from build123d import *

# Parameters (mm, degrees)
SKETCH1_W           = 19.8
SKETCH1_H           = 28
BOSS_EXTRUDE1_DEPTH = 3.7
SKETCH2_W           = 19.8
SKETCH2_H           = 3.7
BOSS_EXTRUDE2_DEPTH = 24.3
CUT_EXTRUDE1_DEPTH  = 9
BOSS_EXTRUDE3_DEPTH = 3.3
BOSS_EXTRUDE4_DEPTH = 3.3
BOSS_EXTRUDE5_DEPTH = 2.1
BOSS_EXTRUDE6_DEPTH = 1.5


with BuildPart() as part:
    # Sketch1 → Boss-Extrude1 (new body)
    with BuildSketch(Plane.XY):
        with Locations((9.9, 14)):
            Rectangle(SKETCH1_W, SKETCH1_H)
        with BuildLine():
            Line((13.2, 15.7), (13.2, 12.3))
            ThreePointArc((13.2, 12.3), (9.9, 9), (6.6, 12.3))
            Line((6.6, 12.3), (6.6, 15.7))
            ThreePointArc((6.6, 15.7), (9.9, 19), (13.2, 15.7))
        make_face(mode=Mode.SUBTRACT)
    extrude(amount=BOSS_EXTRUDE1_DEPTH)

    # Sketch2 → Boss-Extrude2 (add)
    with BuildSketch(Plane.XY.offset(3.7)):
        with Locations((9.9, 1.85)):
            Rectangle(SKETCH2_W, SKETCH2_H)
    extrude(amount=BOSS_EXTRUDE2_DEPTH)

    # Sketch3 → Cut-Extrude1 (cut)
    with BuildSketch(Plane(origin=(0, 3.7, 0), x_dir=(1, 0, 0), z_dir=(0, 1, 0))):
        with BuildLine():
            Line((13.2, -12.3), (13.2, -15.7))
            ThreePointArc((13.2, -15.7), (9.9, -19), (6.6, -15.7))
            Line((6.6, -15.7), (6.6, -12.3))
            ThreePointArc((6.6, -12.3), (9.9, -9), (13.2, -12.3))
        make_face()
    extrude(amount=-CUT_EXTRUDE1_DEPTH, mode=Mode.SUBTRACT)

    # Sketch4 → Boss-Extrude3 (add)
    with BuildSketch(Plane(origin=(19.8, 0, 0), x_dir=(0, 0, -1), z_dir=(1, 0, 0))):
        Polygon((-3.7, 26.4), (-3.7, 3.7), (-26.4, 3.7), (-28, 3.7), (-28, 5.7), (-26.4, 5.7), (-5.7, 26.4), (-5.7, 28), (-3.7, 28), align=None)
    extrude(amount=-BOSS_EXTRUDE3_DEPTH)

    # Sketch5 → Boss-Extrude4 (add)
    with BuildSketch(Plane.ZY):
        Polygon((3.7, 26), (3.7, 3.7), (26, 3.7), (28, 3.7), (28, 5.7), (26.4, 5.7), (5.7, 26.4), (5.7, 28), (3.7, 28), align=None)
    extrude(amount=-BOSS_EXTRUDE4_DEPTH)

    # Sketch6 → Boss-Extrude5 (add)
    with BuildSketch(Plane(origin=(0, 0, 0), x_dir=(-1, 0, 0), z_dir=(0, -1, 0))):
        with BuildLine():
            Line((-9.3, -25.5), (-10.5, -25.5))
            ThreePointArc((-10.5, -25.5), (-12.1, -23.9), (-10.5, -22.3))
            Line((-10.5, -22.3), (-9.3, -22.3))
            ThreePointArc((-9.3, -22.3), (-7.7, -23.9), (-9.3, -25.5))
        make_face()
        with BuildLine():
            Line((-9.45, -4.2), (-10.35, -4.2))
            ThreePointArc((-10.35, -4.2), (-12.1, -2.45), (-10.35, -0.7))
            Line((-10.35, -0.7), (-9.45, -0.7))
            ThreePointArc((-9.45, -0.7), (-7.7, -2.45), (-9.45, -4.2))
        make_face()
    extrude(amount=BOSS_EXTRUDE5_DEPTH)

    # Sketch7 → Boss-Extrude6 (add)
    with BuildSketch(Plane(origin=(0, 0, 0), x_dir=(-1, 0, 0), z_dir=(0, 0, -1))):
        with BuildLine():
            Line((-10.5, 25.5), (-9.3, 25.5))
            ThreePointArc((-9.3, 25.5), (-7.7, 23.9), (-9.3, 22.3))
            Line((-9.3, 22.3), (-10.5, 22.3))
            ThreePointArc((-10.5, 22.3), (-12.1, 23.9), (-10.5, 25.5))
        make_face()
        with BuildLine():
            Line((-10.35, 4.2), (-9.45, 4.2))
            ThreePointArc((-9.45, 4.2), (-7.7, 2.45), (-9.45, 0.7))
            Line((-9.45, 0.7), (-10.35, 0.7))
            ThreePointArc((-10.35, 0.7), (-12.1, 2.45), (-10.35, 4.2))
        make_face()
    extrude(amount=BOSS_EXTRUDE6_DEPTH)


solid = part.part
Verification items for the finished model (mm, model axes). A direction names the side the tool comes from. Coordinates: 2 decimals unless noted, no trailing zeros. Order: outer loops, then holes, each group sorted by start corner. A loop starts at its lowest first (then second) coordinate and runs counter-clockwise, first axis right, second up. Notation, with made-up numbers: M 45.25,35.5 L 101.25,35.5 A27 ccw 101.25,72.5 Z; hole C 7.25,-33 d9. An arc over 180 degrees is marked long. One line per item, written item: value. Start each with the question number.
Item 1: Sectioned sample at C-C on y = 2.45. Record the cut outline in (x, z), then the cut area to 3 significant figures.
Item 2: Access from +Z, -Z, +X, -X, +Y, -Y to the whole of each face (thin tool, end or side, straight path). Record for faces 1 (the cylindrical face through (7.7, 2.5, -0.7)), 2 (the cylindrical face through (12.1, -1, 23.9)), 3 (the cylindrical face through (10, 2, 9)), 4 (the flat face through (13.2, 14, 2)).
Item 3: Sectioned sample at A-A on y = 14. Record the cut outline in (x, z), then the cut area to 3 significant figures.
Item 4: Depth check by flat-ended pin: P1, Ø0.5, axis at x = 9.5, y = -1, coming from the +Z side; P2, Ø0.5, axis at x = 9.5, y = -1, coming from the -Z side; P3, Ø10, axis at x = 9, y = 14.5, coming from the +Z side. Enter the tip coordinate at first touch or a pass-through.
Item 5: Sectioned sample at B-B on x = 9.9. Give the number of separate pieces and of enclosed holes in the cut face, then the cut area to 3 significant figures.
Item 6: Mould release check, pull along Y, two halves, no side actions. Record for faces 5 (the cylindrical face through (10, 9, 2)), 6 (the flat face through (10, 25.5, -1)), 7 (the flat face through (6.6, 2, 14)): pulls with the +Y half, pulls with the -Y half, needs draft (parallel to the pull), parting line crosses it, or undercut.
Item 7: Thickness scan on probe 1 along X at (y, z) = (15.5, 15); probe 2 along Y at (x, z) = (11.75, 26). Record the ranges inside material, lowest first.
Item 8: Sectioned sample at D-D on z = 23.9. Record the cut outline in (x, y).
Calculated:
1. outline: M 0,0 L 7.7,0 L 7.7,-1.5 L 12.1,-1.5 L 12.1,0 L 19.8,0 L 19.8,28 L 0,28 Z; hole M 6.6,12.3 A3.3 ccw 13.2,12.3 L 13.2,15.7 A3.3 ccw 6.6,15.7 Z
1. area: 504 mm^2
2. face 1: -Z, -X
2. face 2: +X, -Y
2. face 3: +Y, -Y
2. face 4: +Z, -Z
3. outline: M 0,0 L 6.6,0 L 6.6,3.7 L 3.3,3.7 L 3.3,18.1 L 0,18.1 Z; M 13.2,0 L 19.8,0 L 19.8,18.1 L 16.5,18.1 L 16.5,3.7 L 13.2,3.7 Z
3. area: 144 mm^2
4. P1: z = 25.5
4. P2: z = 0.7
4. P3: z = 3.7
5. separate pieces: 3
5. enclosed holes: 0
5. area: 144 mm^2
6. face 5: undercut
6. face 6: pulls with the +Y half
6. face 7: needs draft
7. probe 1: 0 to 3.3, 16.5 to 19.8
7. probe 2: 0 to 3.7
8. outline: M 0,0 L 7.7,0 L 7.7,-2.1 L 12.1,-2.1 L 12.1,0 L 19.8,0 L 19.8,8.2 L 16.5,8.2 L 16.5,3.7 L 3.3,3.7 L 3.3,8.2 L 0,8.2 Z
